from build123d import *

# Parameters (mm, degrees)
CHANFREIN1_SIZE         = 0.2
ESQUISSE3_W             = 8
ESQUISSE3_H             = 2
ENL_V_MAT_EXTRU_2_DEPTH = 8
ESQUISSE4_W             = 3
ESQUISSE4_H             = 8
ENL_V_MAT_EXTRU_3_DEPTH = 10


with BuildPart() as part:
    # Esquisse1 → Révolution1 (revolve)
    with BuildSketch(Plane.XY, mode=Mode.PRIVATE) as r_volution1_sk:
        Polygon((-4.5, 6), (-13, 6), (-13, 3), (-22, 3), (-22, 0), (0, 0), (0, 8), (-4.5, 8), align=None)
    revolve(r_volution1_sk.sketch.rotate(Axis((0, 0, 0), (1, 0, 0)), 90), axis=Axis((0, 0, 0), (1, 0, 0)))

    # Chanfrein1
    chanfrein1_edges = [part.edges().sort_by_distance(p)[0] for p in [
        (0, 0, -8),
        (-4.5, 0, -8),
        (-13, 0, -6),
        (-22, 0, -3),
    ]]
    chamfer(chanfrein1_edges, length=CHANFREIN1_SIZE)

    # Esquisse3 → Enlèv. mat.-Extru.2 (cut)
    with BuildSketch(Plane.ZY.offset(22)):
        with Locations((0, 3.5)):
            Rectangle(ESQUISSE3_W, ESQUISSE3_H)
    extrude(amount=-ENL_V_MAT_EXTRU_2_DEPTH, mode=Mode.SUBTRACT)

    # Esquisse4 → Enlèv. mat.-Extru.3 (cut, symmetric)
    with BuildSketch(Plane.XY):
        with Locations((-1.5, 0)):
            Rectangle(ESQUISSE4_W, ESQUISSE4_H)
    extrude(amount=ENL_V_MAT_EXTRU_3_DEPTH, both=True, mode=Mode.SUBTRACT)


solid = part.part
Design review of the part built by this model. Coordinates are the model's own, in mm. A direction names the side the tool comes from. Give positions to 0.01 mm unless a question says otherwise; leave off trailing zeros. Order: outer loops, then holes, each group sorted by start corner. A loop starts at its lowest first (then second) coordinate and runs counter-clockwise, first axis right, second up. Notation, with made-up numbers: (24.5, 79) - (42.5, 79) arc R21 ccw to (42.5, 91) - close; hole circle Ø5 at (-13, -19.75). An arc over 180 degrees is marked (long way). Write item = value, one per line. Start each with the question number.
Q1. We need section C-C on x = -8.5. State the section outline as (y, z) points.
Q2. To check wall thickness, follow L1, parallel to X at y = 0.5, z = 0; L2, parallel to X at y = 1.25, z = -4.75; L3, parallel to Y at x = -12.75, z = -2.25. State the ranges of each line that lie inside material, in increasing order. Write a range as from..to.
Q3. We need section A-A on z = 0. State the section outline as (x, y) points.
Q4. We need section D-D on x = -20.5. State the section outline as (y, z) points.
Q5. Mouldability with a two-part tool opening along Y and no side actions: class faces 1 (the face through (-13, 2.5, 2.5)), 2 (the face through (-3.19, -0.352, -7.992)), 3 (the face through (-3, 0, 0)) as released by +Y, released by -Y, zero draft, split by the parting line, or undercut.
Q6. Clearance check with flat-ended pins moving along their axes: pin 1 Ø6 at (x, y) = (-17.5, -4.5) entering from +Z; pin 2 Ø1.5 at (y, z) = (5.5, -6.5) entering from -X; pin 3 Ø1.5 at (x, z) = (-9.5, -0.5) entering from +Y. State where each tip first meets the part, or that it passes through.
Q7. We need section B-B on y = 0. State the section outline as (x, z) points.
Q8. Tool access review of faces 4 (the face through (-22, 0, 0)), 5 (the face through (-18, 2.5, 0)), 6 (the face through (0, -6, 0)), 7 (the face through (-17, -3, 0)), 8 (the face through (-2, -4, 0)): name each direction out of +Z, -Z, +X, -X, +Y, -Y from which nothing blocks a thin tool from reaching the whole face with its end or side.
Working result:
q1.outline = circle Ø12 at (0, 0)
q2.L1 = -22..-3
q2.L2 = -13..-3
q2.L3 = -5.56..5.56
q3.outline = (-22, -2.8) - (-21.8, -3) - (-13, -3) - (-13, -5.8) - (-12.8, -6) - (-4.5, -6) - (-4.5, -7.8) - (-4.3, -8) - (-0.2, -8) - (0, -7.8) - (0, -4) - (-3, -4) - (-3, 4) - (0, 4) - (0, 7.8) - (-0.2, 8) - (-4.3, 8) - (-4.5, 7.8) - (-4.5, 6) - (-12.8, 6) - (-13, 5.8) - (-13, 3) - (-14, 3) - (-14, 2.5) - (-22, 2.5) - close
q4.outline = (2.5, -1.66) - (2.5, 1.66) arc R3 ccw (long way) to start
q5.face_1 = zero draft
q5.face_2 = split by the parting line
q5.face_3 = undercut
q6.pin_1 = 2.6
q6.pin_2 = -4.5
q6.pin_3 = 6
q7.outline = (-22, -2.8) - (-21.8, -3) - (-13, -3) - (-13, -5.8) - (-12.8, -6) - (-4.5, -6) - (-4.5, -7.8) - (-4.3, -8) - (-3, -8) - (-3, 8) - (-4.3, 8) - (-4.5, 7.8) - (-4.5, 6) - (-12.8, 6) - (-13, 5.8) - (-13, 3) - (-21.8, 3) - (-22, 2.8) - close
q8.face_4 = +Z, -Z, -X, +Y, -Y
q8.face_5 = +Z, -Z, -X, +Y
q8.face_6 = +Z, -Z, +X, +Y, -Y
q8.face_7 = -X
q8.face_8 = +Z, -Z, +X
